from build123d import *

# Parameters (mm, degrees)
F1_DEPTH = 162.5


with BuildPart() as f1:
    # F0 (on Front) → F1 (new body, symmetric)
    with BuildSketch(Plane.XZ):
        Polygon((-4.775, 10), (-10, 10), (-10, 4.775), (-8.325, 3.1), (-8.325, 5.5), (-6.6844038585, 5.5), (-3.75, 2.5655961415), (-3.75, 0), (-3.75, -2.5655961415), (-6.6844038585, -5.5), (-8.325, -5.5), (-8.325, -3.1), (-10, -4.775), (-10, -10), (-4.775, -10), (-3.1, -8.325), (-5.5, -8.325), (-5.5, -6.6844038585), (-2.5655961415, -3.75), (0, -3.75), (2.5655961415, -3.75), (5.5, -6.6844038585), (5.5, -8.325), (3.1, -8.325), (4.775, -10), (10, -10), (10, -4.775), (8.325, -3.1), (8.325, -5.5), (6.6844038585, -5.5), (3.75, -2.5655961415), (3.75, 0), (3.75, 2.5655961415), (6.6844038585, 5.5), (8.325, 5.5), (8.325, 3.1), (10, 4.775), (10, 10), (4.775, 10), (3.1, 8.325), (5.5, 8.325), (5.5, 6.6844038585), (2.5655961415, 3.75), (0, 3.75), (-2.5655961415, 3.75), (-5.5, 6.6844038585), (-5.5, 8.325), (-3.1, 8.325), align=None)
    extrude(amount=F1_DEPTH, both=True)


solid = f1.part
Geometry check sheet. Reference: the model listing, model coordinates, mm. A direction names the side the tool comes from. Round coordinates to 2 decimals unless told otherwise and drop trailing zeros.
Item 1: Gauge pin test, flat ends, axial feed: pin 1 (5.5 mm diameter, centred on x = 1, y = 36, fed in from -Z) (3 decimals); pin 2 (1 mm diameter, centred on x = -0.5, y = -100.5, fed in from +Z); pin 3 (1.5 mm diameter, centred on y = -53.5, z = 0.5, fed in from +X); pin 4 (2 mm diameter, centred on x = -7, z = 1.5, fed in from +Y). Record the tip position at first contact, or that the pin passes through.
Item 2: Mould release check, pull along Z, two halves, no side actions. Record for faces 4 (the flat face through (-7, -2, -10)), 5 (the flat face through (3.75, -2, 0)), 6 (the flat face through (-10, -2, -7)), 7 (the flat face through (-3.75, -2, 0)): pulls with the +Z half, pulls with the -Z half, needs draft (parallel to the pull), parting line crosses it, or undercut.
Item 3: Access from +Z, -Z, +X, -X, +Y, -Y to the whole of each face (thin tool, end or side, straight path). Record for faces 1 (the flat face through (0, -2, 3.75)), 2 (the flat face through (10, -2, -7)), 3 (the flat face through (0, -2, -3.75)).
Item 4: Thickness scan on line 1 (X direction, y = -32, z = 6.75); line 2 (X direction, y = 62.5, z = -4.5) (3 decimals); line 3 (Z direction, x = -4.75, y = 9.5) (3 decimals). Record the ranges inside material, lowest first.
Answer sheet:
1. pin 1: stops at z = -8.975
1. pin 2: stops at z = 3.75
1. pin 3: stops at x = 3.75
1. pin 4: passes through
2. face 4: pulls with the -Z half
2. face 5: undercut
2. face 6: needs draft
2. face 7: undercut
3. face 1: +Z, +Y, -Y
3. face 2: +Z, -Z, +X, +Y, -Y
3. face 3: -Z, +Y, -Y
4. line 1: x = -10 to -5.5, 5.5 to 10
4. line 2: x = -9.725 to -8.325, -5.684 to -3.316, 3.316 to 5.684, 8.325 to 9.725
4. line 3: z = -9.975 to -8.325, -5.934 to -3.566, 3.566 to 5.934, 8.325 to 9.975
